from build123d import *

# Parameters (mm, degrees)
CROQUIS1_R              = 19.15
SALIENTE_EXTRUIR1_DEPTH = 34.82
CROQUIS2_R              = 9.975
SALIENTE_EXTRUIR2_DEPTH = 4.95
SALIENTE_EXTRUIR3_DEPTH = 12
CROQUIS4_R              = 4.865
SALIENTE_EXTRUIR4_DEPTH = 20
CROQUIS5_R              = 19.25
SALIENTE_EXTRUIR5_DEPTH = 2
CROQUIS6_R              = 1.5
CORTAR_EXTRUIR1_DEPTH   = 5


with BuildPart() as part:
    # Croquis1 → Saliente-Extruir1 (new body)
    with BuildSketch(Plane.XY):
        Circle(CROQUIS1_R)
    extrude(amount=SALIENTE_EXTRUIR1_DEPTH)

    # Croquis2 → Saliente-Extruir2 (add)
    with BuildSketch(Plane(origin=(0, 0, 0), x_dir=(-1, 0, 0), z_dir=(0, 0, -1))):
        with Locations(Location((0, 0, 0), (0, 0, 180))):
            Circle(CROQUIS2_R)
    extrude(amount=SALIENTE_EXTRUIR2_DEPTH)

    # Croquis3 → Saliente-Extruir3 (add)
    with BuildSketch(Plane(origin=(0, 0, -4.95), x_dir=(-1, 0, 0), z_dir=(0, 0, -1))):
        with BuildLine():
            Line((-1.839320527, -2.37), (1.839320527, -2.37))
            ThreePointArc((1.839320527, -2.37), (0, 3), (-1.839320527, -2.37))
        make_face()
    extrude(amount=SALIENTE_EXTRUIR3_DEPTH)

    # Croquis4 → Saliente-Extruir4 (add)
    with BuildSketch(Plane(origin=(0, 0, 0), x_dir=(1, 0, 0), z_dir=(0, 1, 0))):
        with Locations(Location((0, -29.955, 0), (0, 0, 270))):
            Circle(CROQUIS4_R)
    extrude(amount=SALIENTE_EXTRUIR4_DEPTH)

    # Croquis5 → Saliente-Extruir5 (add)
    with BuildSketch(Plane(origin=(0, 0, 0), x_dir=(-1, 0, 0), z_dir=(0, 0, -1))):
        Circle(CROQUIS5_R)
    extrude(amount=-SALIENTE_EXTRUIR5_DEPTH)

    # Croquis6 → Cortar-Extruir1 (cut)
    with BuildSketch(Plane(origin=(0, 0, 0), x_dir=(-1, 0, 0), z_dir=(0, 0, -1))):
        with Locations((-10.962942032, 9.38867591)):
            Circle(CROQUIS6_R)
        with Locations((13.612302862, 4.799848345)):
            Circle(CROQUIS6_R)
        with Locations((-2.64936083, -14.188524255)):
            Circle(CROQUIS6_R)
    extrude(amount=-CORTAR_EXTRUIR1_DEPTH, mode=Mode.SUBTRACT)


solid = part.part
Design review of the part built by this model. Coordinates are the model's own, in mm. A direction names the side the tool comes from. Coordinates: 2 decimals unless noted, no trailing zeros. Loops run counter-clockwise (first coordinate to the right, second up) from the corner with the lowest first, then second, coordinate; pieces in that order, holes last. Notation, with made-up numbers: M -25,52.25 L 2,52.25 A20 cw 2,60.25 Z; hole C 67.5,9.5 d3. An arc over 180 degrees is marked long. Use one line per item in the form item = value.
(1) Consider section C-C (z = 3.5). Write out the cut boundary in (x, y), and give its area (3 significant figures).
Return value:
outline = C 0,0 d38.3; hole C -13.61,4.8 d3; hole C 2.65,-14.19 d3; hole C 10.96,9.39 d3
area = 1,130 mm2
(2) For line 1 along Z through (x, y) = (15, -0.5); line 2 along Z through (x, y) = (5.5, 3); line 3 along X through (y, z) = (-8, 7), list the stretches that pass through material, from the lowest coordinate up. Write a range as from..to.
Return value:
line_1 = 0..34.82
line_2 = -4.95..34.82
line_3 = -17.4..17.4
(3) Consider section A-A (y = 0). Write out the cut boundary in (x, z) (3 decimals).
Return value:
outline = M -19.25,0 L -9.975,0 L -9.975,-4.95 L -3,-4.95 L -3,-16.95 L 3,-16.95 L 3,-4.95 L 9.975,-4.95 L 9.975,0 L 19.25,0 L 19.25,2 L 19.15,2 L 19.15,34.82 L -19.15,34.82 L -19.15,2 L -19.25,2 Z
(4) Clearance check with flat-ended pins moving along their axes: P1, Ø5, axis at y = 13, z = 16, coming from the -X side; P2, Ø2.5, axis at x = 11, y = 9.5, coming from the -Z side; P3, Ø1.5, axis at x = -1, z = 19.5, coming from the +Y side. State where each tip first meets the part, or that it passes through.
Return value:
P1 = -16.01
P2 = 5
P3 = 19.15
(5) Consider section D-D (z = -12). Write out the cut boundary in (x, y), and give its area (3 significant figures).
Return value:
outline = M -1.84,-2.37 L 1.84,-2.37 A3 ccw long Z
area = 26.7 mm2
(6) For faces 4 (the face through (0, 0, -16.95)), 5 (the face through (-2.96, 19.414, 26.094)), 6 (the face through (11, 9, 5)), list the 3-axis set-ups (+Z, -Z, +X, -X, +Y, -Y) from which the entire face can be reached by the end or side of a thin tool; tool diameter is ignored.
Return value:
face_4 = -Z, +X, -X, +Y, -Y
face_5 = +Y
face_6 = -Z
(7) Consider section B-B (z = 16). Write out the cut boundary in (x, y), and give its area (3 significant figures).
Return value:
outline = C 0,0 d38.3
area = 1,150 mm2
(8) Draft analysis for pull direction X (two halves, no side actions). For faces 1 (the face through (0, -2.37, -11)), 2 (the face through (3, -14, 5)), 3 (the face through (9.514, -2.996, -2.44)), state which applies: pulls with the +X half, pulls with the -X half, needs draft (parallel to the pull), parting line crosses it, or undercut.
Return value:
face_1 = needs draft
face_2 = undercut
face_3 = parting line crosses it
